For this review, take the finished solid that the model builds, in its own axes (mm). Coordinates: 2 decimals unless noted, no trailing zeros. Loops run counter-clockwise (first coordinate to the right, second up) from the corner with the lowest first, then second, coordinate; pieces in that order, holes last. Notation, with made-up numbers: (82, 35) - (128, 35) arc R19 ccw to (128, 45) - close; hole circle Ø11 at (87.5, 30). An arc over 180 degrees is marked (long way). Answer as a JSON object with one key per item and string values. Group by question number.
Item 1: Mouldability with a two-part tool opening along X and no side actions: class faces 1 (the cylindrical face through (-0.07, 1.75, -19.15)), 2 (the flat face through (0, 0, 0)), 3 (the cylindrical face through (5.506, 0.986, 24.796)) as released by +X, released by -X, zero draft, split by the parting line, or undercut.
Item 2: We need section D-D (z = 6.5). Give the boundary of the cut face in (x, y).
Item 3: We need section C-C (x = 10). Give the boundary of the cut face in (y, z).
Item 4: Clearance check with flat-ended pins moving along their axes: pin 1 (1 mm diameter, centred on y = 1.5, z = 18, fed in from -X); pin 2 (1 mm diameter, centred on y = 1.5, z = 16, fed in from +X); pin 3 (2.5 mm diameter, centred on x = -20.65, z = 0, fed in from +Y). State where each tip first meets the part, or that it passes through.
Item 5: We need section A-A (x = 0). Give the boundary of the cut face in (y, z), then the cut area to 3 significant figures.
Item 6: To check wall thickness, follow line 1 (Z direction, x = 0, y = 1.7); line 2 (Z direction, x = -2.5, y = 1.3); line 3 (Z direction, x = -20.5, y = 0.7). State the ranges of each line that lie inside material, in increasing order.
Item 7: We need section B-B (z = 0). Give the boundary of the cut face in (x, y).
Autodesk Inventor part; units mm, degrees
ref_plane "YZ Plane" through (0, 0, 0) normal (1, 0, 0) x (0, 1, 0)
ref_plane "XZ Plane" through (0, 0, 0) normal (0, 1, 0) x (-1, 0, 0)
ref_plane "XY Plane" through (0, 0, 0) normal (0, 0, 1) x (1, 0, 0)
sketch "Skizze1" plane through (0, 0, 0) normal (0, 1, 0) x (-1, 0, 0)
  circle A0 centre (0, 0) radius 25.4
  dimension "d0" = 50.8
extrude "Extrusion1" add sketch "Skizze1" along normal blind 2
sketch "Skizze2" plane through (0, 0, 0) normal (0, -1, 0) x (1, 0, 0)
  circle A0 centre (0, 0) radius 25.4
  line L0 (-20.6475, 0) -> (0, 20.6475) construction
  line L1 (0, 20.6475) -> (20.6475, 0) construction
  line L2 (20.6475, 0) -> (0, -20.6475) construction
  line L3 (0, -20.6475) -> (-20.6475, 0) construction
  line L4 (0, 0) -> (10.3238, 10.3238) construction
  line L5 (0, 0) -> (-10.3238, 10.3238) construction
  circle A1 centre (0, 0) radius 25.4 construction
  line L6 (0, 0) -> (0, 25.4) construction
  point P0 (-20.6475, 0)
  point P1 (0, 20.6475)
  point P2 (20.6475, 0)
  dimension "d3" = 29.2
  dimension "d4" = 29.2
  dimension "d63" = 45
hole "Bohrung1" at (-20.6475, 0, 0) at (0, 0, 20.6475) at (20.6475, 0, 0) at (0, 0, -20.6475) direction (0, 1, 0) diameter 3 end through all countersink diameter 6 countersink angle 90
sketch "Skizze7" plane through (0, 0, 0) normal (0, -1, 0) x (1, 0, 0)
  circle A0 centre (0, 0) radius 25.4 construction
  circle A1 centre (0, 0) radius 10 construction
  line L0 (0, 0) -> (10, 0) construction
  circle A2 centre (0, 0) radius 10 construction
  line L1 (0, 0) -> (-5, 8.6603) construction
  circle A3 centre (0, 0) radius 10 construction
  line L2 (0, 0) -> (-5, -8.6603) construction
  dimension "d68" = 20
  dimension "d71" = 360
hole "Bohrung3" at (-5, 0, 8.6603) at (10, 0, 0) at (-5, 0, -8.6603) direction (0, 1, 0) diameter 7 end through all
properties part number "anschluss_daten"
Check sheet entries:
{
 "1": {"face 1": "undercut", "face 2": "zero draft", "face 3": "split by the parting line"},
 "2": {"outline": "(-24.55, 0) - (-7.75, 0) - (-7.75, 2) - (-24.55, 2) - close; (-2.25, 0) - (24.55, 0) - (24.55, 2) - (-2.25, 2) - close"},
 "3": {"outline": "(0, -23.35) - (2, -23.35) - (2, -3.5) - (0, -3.5) - close; (0, 3.5) - (2, 3.5) - (2, 23.35) - (0, 23.35) - close"},
 "4": {"pin 1": "stops at x = -18.41", "pin 2": "stops at x = 20.12", "pin 3": "passes through"},
 "5": {"outline": "(0, -25.4) - (2, -25.4) - (2, -22.15) - (1.5, -22.15) - (0, -23.65) - close; (0, -17.65) - (1.5, -19.15) - (2, -19.15) - (2, 19.15) - (1.5, 19.15) - (0, 17.65) - close; (0, 23.65) - (1.5, 22.15) - (2, 22.15) - (2, 25.4) - (0, 25.4) - close", "area": "85.1 mm2"},
 "6": {"line 1": "z = -25.4 to -22.15, -19.15 to 19.15, 22.15 to 25.4", "line 2": "z = -25.28 to -11.11, -6.21 to 6.21, 11.11 to 25.28", "line 3": "z = -15 to -2.3, 2.3 to 15"},
 "7": {"outline": "(-25.4, 0) - (-23.65, 0) - (-22.15, 1.5) - (-22.15, 2) - (-25.4, 2) - close; (-19.15, 1.5) - (-17.65, 0) - (6.5, 0) - (6.5, 2) - (-19.15, 2) - close; (13.5, 0) - (17.65, 0) - (19.15, 1.5) - (19.15, 2) - (13.5, 2) - close; (22.15, 1.5) - (23.65, 0) - (25.4, 0) - (25.4, 2) - (22.15, 2) - close"}
}
